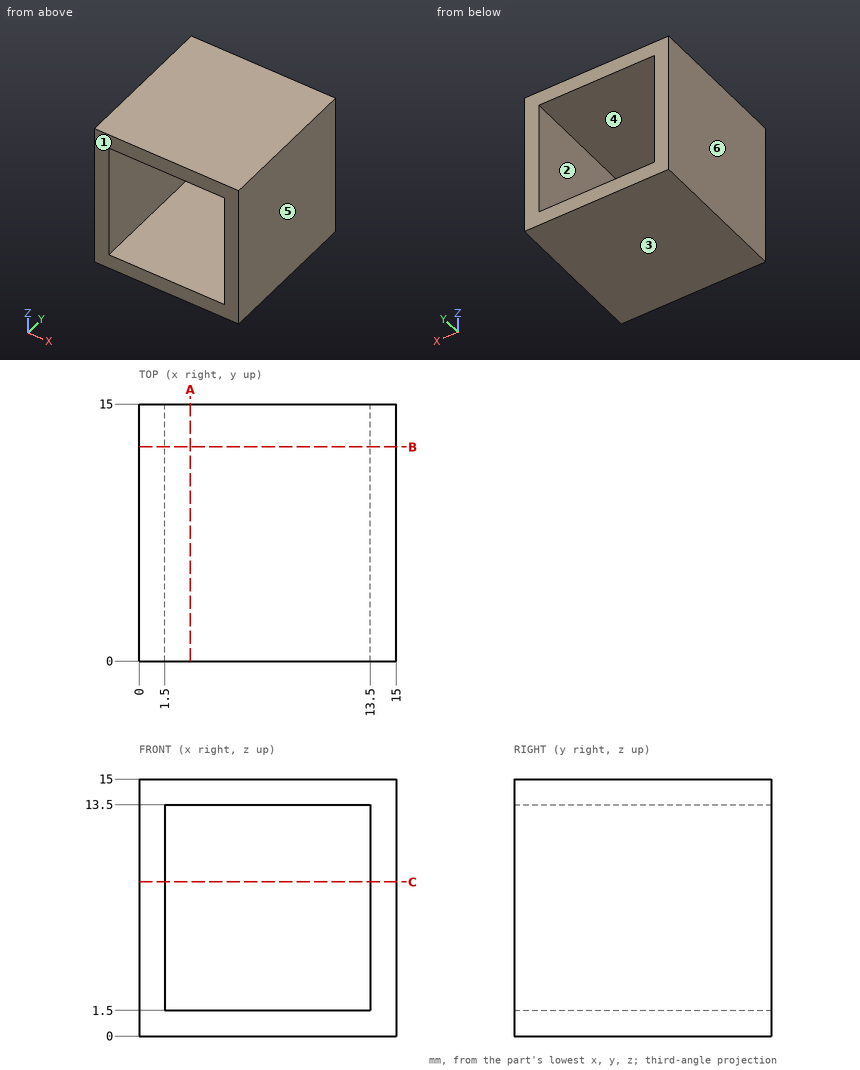
Design review of the part shown in the three views and the two pictorial views. Dimensions are in mm from the part's minimum x, y and z. A direction names the side the tool comes from. Give positions to 0.01 mm unless a question says otherwise; leave off trailing zeros. Loops run counter-clockwise (first coordinate to the right, second up) from the corner with the lowest first, then second, coordinate; pieces in that order, holes last. Notation, with made-up numbers: (13.25, 49.5) - (45.25, 49.5) arc R29 ccw to (45.25, 78.5) - close; hole circle Ø1 at (30, 16.25). An arc over 180 degrees is marked (long way). Answer as a JSON object with one key per item and string values.
Q1. Add section B-B on y = 12.5. State the section outline as (x, z) points, plus the area to 3 significant figures.
Worked out:
{"outline": "(0, 0) - (15, 0) - (15, 15) - (0, 15) - close; hole (1.5, 1.5) - (13.5, 1.5) - (13.5, 13.5) - (1.5, 13.5) - close", "area": "81.0 mm^2"}
Q2. Add section A-A on x = 3. State the section outline as (y, z) points.
Worked out:
{"outline": "(0, 0) - (15, 0) - (15, 1.5) - (0, 1.5) - close; (0, 13.5) - (15, 13.5) - (15, 15) - (0, 15) - close"}
Q3. For the marked faces 1 and 2, list the 3-axis set-ups (+Z, -Z, +X, -X, +Y, -Y) from which the entire face can be reached by the end or side of a thin tool; tool diameter is ignored.
Worked out:
{"face 1": "+Z, -Z, +X, -X, -Y", "face 2": "+Y, -Y"}
Q4. Insertion check: pin 1 (4 mm diameter, centred on x = 8.5, z = 10.5, fed in from -Y). The pin has a flat end and moves straight along its axis. Give the tip position at first contact, or say it passes through.
Worked out:
{"pin 1": "passes through"}
Q5. Mouldability with a two-part tool opening along X and no side actions: class the marked faces 3, 4, 5 and 6 as +X half, -X half, draft (parallel to the pull), parting line (faces both ways), or undercut.
Worked out:
{"face 3": "draft", "face 4": "undercut", "face 5": "+X half", "face 6": "-X half"}
Q6. Add section C-C on z = 9. State the section outline as (x, y) points, plus the area to 3 significant figures.
Worked out:
{"outline": "(0, 0) - (1.5, 0) - (1.5, 15) - (0, 15) - close; (13.5, 0) - (15, 0) - (15, 15) - (13.5, 15) - close", "area": "45.0 mm^2"}
Q7. To check wall thickness, follow line 1 along Z through (x, y) = (12, 13.75). State the ranges of the line that lie inside material, in increasing order.
Worked out:
{"line 1": "z = 0 to 1.5, 13.5 to 15"}
